```python
from build123d import *

# Parameters (mm, degrees)
EXTRUDE_1_DEPTH     = 81
SKETCH_2_R          = 2.25
CUT_EXTRUDE_1_DEPTH = 82
SKETCH_3_R          = 1.75
CUT_EXTRUDE_2_DEPTH = 82
FILLET_1_R          = 10
FILLET_3_R          = 15
SKETCH_6_W          = 13
SKETCH_6_H          = 29
CUT_EXTRUDE_3_DEPTH = 55
FILLET_4_R          = 4


with BuildPart() as part:
    # 草图1 → 凸台-拉伸1 (new body)
    with BuildSketch(Plane.XY):
        Polygon((18.05, -15), (10.5, -15), (10.5, -51), (21, -51), (21, 0), (18.05, 0), align=None)
        Polygon((10.5, -51), (10.5, -15), (2.95, -15), (2.95, 0), (0, 0), (0, -51), align=None)
    extrude(amount=EXTRUDE_1_DEPTH)

    # 草图2 → 切除-拉伸1 (cut)
    with BuildSketch(Plane.XZ.offset(51)):
        with Locations(Location((10.5, 20.5, 0), (0, 0, 270))):
            Circle(SKETCH_2_R)
        with Locations(Location((10.5, 60.5, 0), (0, 0, 270))):
            Circle(SKETCH_2_R)
    extrude(amount=-CUT_EXTRUDE_1_DEPTH, mode=Mode.SUBTRACT)

    # 草图3 → 切除-拉伸2 (cut)
    with BuildSketch(Plane(origin=(21, 0, 0), x_dir=(0, 0, -1), z_dir=(1, 0, 0))):
        with Locations(Location((-70.5, -42.25, 0), (0, 0, 90))):
            Circle(SKETCH_3_R)
        with Locations(Location((-10.5, -42.25, 0), (0, 0, 90))):
            Circle(SKETCH_3_R)
    extrude(amount=-CUT_EXTRUDE_2_DEPTH, mode=Mode.SUBTRACT)

    # 圆角1
    fillet_1_edges = [part.edges().sort_by_distance(p)[0] for p in [
        (19.525, 0, 0),
        (1.475, 0, 0),
        (1.475, 0, 81),
        (19.525, 0, 81),
    ]]
    fillet(fillet_1_edges, radius=FILLET_1_R)

    # 圆角3
    fillet_3_edges = [part.edges().sort_by_distance(p)[0] for p in [
        (10.5, -51, 0),
        (10.5, -51, 81),
    ]]
    fillet(fillet_3_edges, radius=FILLET_3_R)

    # 草图6 → 切除-拉伸3 (cut)
    with BuildSketch(Plane(origin=(21, 0, 0), x_dir=(0, 0, -1), z_dir=(1, 0, 0))):
        with Locations((-34, -36.5)):
            Rectangle(SKETCH_6_W, SKETCH_6_H)
        with Locations((-47, -36.5)):
            Rectangle(SKETCH_6_W, SKETCH_6_H)
    extrude(amount=-CUT_EXTRUDE_3_DEPTH, mode=Mode.SUBTRACT)

    # 圆角4
    fillet_4_edges = [part.edges().sort_by_distance(p)[0] for p in [
        (10.5, -22, 53.5),
        (10.5, -22, 27.5),
        (10.5, -51, 27.5),
        (10.5, -51, 53.5),
    ]]
    fillet(fillet_4_edges, radius=FILLET_4_R)


solid = part.part
```
The model under review builds one solid part; all positions refer to its coordinate system, in mm. A direction names the side the tool comes from. Give positions to 0.01 mm unless a question says otherwise; leave off trailing zeros. Write each loop counter-clockwise with the first axis right and the second up, starting at its lowest first coordinate (ties: lowest second). Pieces come first, ordered by that corner, then holes. Notation, with made-up numbers: (-34.5, -33.75) - (11.5, -33.75) arc R23 cw to (11.5, 3.25) - close; hole circle Ø1 at (-27, -36). An arc over 180 degrees is marked (long way). Answer in a Markdown table with one row per item. Add a question column.
1. Draft analysis for pull direction Y (two halves, no side actions). For faces 4 (the cylindrical face through (10.647, -40.633, 69.83)), 5 (the flat face through (11, -15, 40)), 6 (the flat face through (0, -19, 40)), state which applies: +Y half, -Y half, draft (parallel to the pull), parting line (faces both ways), or undercut.
2. We need section D-D on x = 5.25. Write out the cut boundary in (y, z).
3. We need section C-C on y = -37. Write out the cut boundary in (x, z), then the cut area to 3 significant figures.
4. Insertion check: P1, Ø1, axis at x = 18.5, z = 9, coming from the -Y side; P2, Ø3, axis at y = -42.25, z = 10.5, coming from the +X side; P3, Ø6, axis at x = 10.5, z = 20.5, coming from the +Y side. Each pin has a flat end and moves straight along its axis. Give the tip position at first contact, or say it passes through.
5. We need section B-B on z = 20.5. Write out the cut boundary in (x, y).
6. Wall thickness on line 1 along X through (y, z) = (-30.5, 20.5); line 2 along Z through (x, y) = (5.25, -42.25); line 3 along X through (y, z) = (-7, 70.5): over which ranges is each line inside the solid? List them lowest first. Write a range as [from, to].
7. Tool access review of faces 1 (the flat face through (18.05, -7, 40)), 2 (the cylindrical face through (10.353, -23.141, 52.297)), 3 (the cylindrical face through (10.647, -40.581, 11.026)): name each direction out of +Z, -Z, +X, -X, +Y, -Y from which nothing blocks a thin tool from reaching the whole face with its end or side.
8. We need section A-A on x = 10.5. Write out the cut boundary in (y, z), then the cut area to 3 significant figures.
Ans:
| question | item | result |
|---|---|---|
| 1 | face 4 | undercut |
| 1 | face 5 | +Y half |
| 1 | face 6 | draft |
| 2 | outline | (-51, 15) arc R15 ccw to (-36, 0) - (-15, 0) - (-15, 81) - (-36, 81) arc R15 ccw to (-51, 66) - (-51, 57.5) arc R4 ccw to (-47, 53.5) - (-26, 53.5) arc R4 cw to (-22, 49.5) - (-22, 31.5) arc R4 cw to (-26, 27.5) - (-47, 27.5) arc R4 ccw to (-51, 23.5) - close; hole circle Ø3.5 at (-42.25, 10.5); hole circle Ø3.5 at (-42.25, 70.5) |
| 3 | outline | (0, 0.03) - (21, 0.03) - (21, 27.5) - (0, 27.5) - close; (0, 53.5) - (21, 53.5) - (21, 80.97) - (0, 80.97) - close; hole circle Ø4.5 at (10.5, 20.5); hole circle Ø4.5 at (10.5, 60.5) |
| 3 | area | 1,120 mm^2 |
| 4 | P1 | stops at y = -49.96 |
| 4 | P2 | passes through |
| 4 | P3 | stops at y = -15 |
| 5 | outline | (0, -51) - (8.25, -51) - (8.25, -15) - (2.95, -15) - (2.95, 0) - (0, 0) - close; (12.75, -51) - (21, -51) - (21, 0) - (18.05, 0) - (18.05, -15) - (12.75, -15) - close |
| 6 | line 1 | x = [0, 8.25], [12.75, 21] |
| 6 | line 2 | z = [1.36, 8.75], [12.25, 27.5], [53.5, 68.75], [72.25, 79.64] |
| 6 | line 3 | x = [0, 2.95], [18.05, 21] |
| 7 | face 1 | +Z, -Z, +Y |
| 7 | face 2 | +X, -X, -Y |
| 7 | face 3 | +X, -X |
| 8 | outline | (-51, 15) arc R15 ccw to (-36, 0) - (-15, 0) - (-15, 18.25) - (-51, 18.25) - close; (-51, 22.75) - (-15, 22.75) - (-15, 58.25) - (-51, 58.25) - (-51, 57.5) arc R4 ccw to (-47, 53.5) - (-26, 53.5) arc R4 cw to (-22, 49.5) - (-22, 31.5) arc R4 cw to (-26, 27.5) - (-47, 27.5) arc R4 ccw to (-51, 23.5) - close; (-51, 62.75) - (-15, 62.75) - (-15, 81) - (-36, 81) arc R15 ccw to (-51, 66) - close; hole circle Ø3.5 at (-42.25, 10.5); hole circle Ø3.5 at (-42.25, 70.5) |
| 8 | area | 1,720 mm^2 |
